For this review, take the finished solid that the model builds, in its own axes (mm). Face numbers are marked on the shaded views. A direction names the side the tool comes from. Coordinates: 2 decimals unless noted, no trailing zeros. Loops run counter-clockwise (first coordinate to the right, second up) from the corner with the lowest first, then second, coordinate; pieces in that order, holes last. Notation, with made-up numbers: (5.5, 83) -> (14.5, 83) arc R26 cw to (14.5, 98) -> close; hole circle Ø1 at (80, 18.25). An arc over 180 degrees is marked (long way). Use a Markdown table: item, result.
from build123d import *

# Parameters (mm, degrees)
F1_DEPTH = 10
F6_DEPTH = 25


with BuildPart() as f1:
    # F0 (on Top) → F1 (new body)
    with BuildSketch(Plane.XY):
        Polygon((25, 4.25), (25, 0), (30, 0), (30, 7.25), (0, 7.25), (0, 4.25), align=None)
    extrude(amount=F1_DEPTH)

    # F2 (on face) → F3 (revolve)
    with BuildSketch(Plane(origin=(0, 7.25, 0), x_dir=(-1, 0, 0), z_dir=(0, 1, 0))):
        with BuildLine():
            Line((-7.5, 7.25), (-7.5, 2.75))
            ThreePointArc((-7.5, 2.75), (-5.25, 5), (-7.5, 7.25))
        make_face()
    revolve(axis=Axis((7.5, 7.25, 5), (0, 0, -1)))

    # F4: F1 across plane


with BuildPart() as f1_1:
    add(f1.part)
    add(f1.part.mirror(Plane.XZ))

    # F5 (on face) → F6 (cut)
    with BuildSketch(Plane.XZ.offset(7.25)):
        with BuildLine():
            ThreePointArc((7.5, 0), (2.5, 5), (7.5, 10))
            Line((7.5, 10), (0, 10))
            Line((0, 10), (0, 0))
            Line((0, 0), (7.5, 0))
        make_face()
    extrude(amount=-F6_DEPTH, mode=Mode.SUBTRACT)


solid = f1_1.part
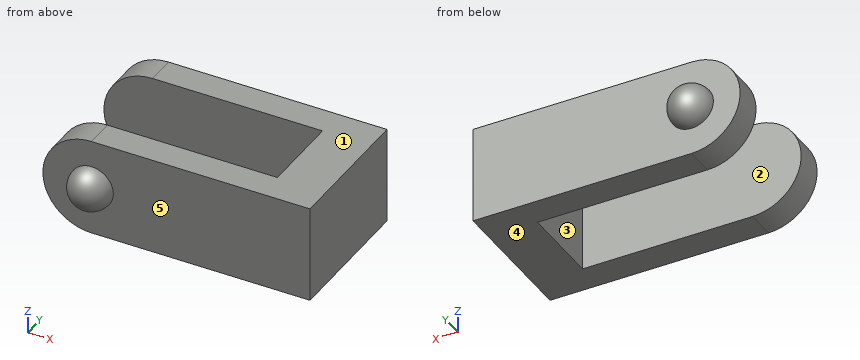
(1) Take a section at B-B on z = 9. Write out the cut boundary in (x, y).
Found:
| item | result |
|---|---|
| outline | (4.5, -7.25) -> (30, -7.25) -> (30, 7.25) -> (4.5, 7.25) -> (4.5, 4.25) -> (25, 4.25) -> (25, -4.25) -> (4.5, -4.25) -> close |
(2) Mouldability with a two-part tool opening along Y and no side actions: class the marked faces 3, 4 and 5 as pulls with the +Y half, pulls with the -Y half, needs draft (parallel to the pull), parting line crosses it, or undercut.
Found:
| item | result |
|---|---|
| face 3 | undercut |
| face 4 | needs draft |
| face 5 | pulls with the -Y half |
(3) Take a section at D-D on y = 2.75. Write out the cut boundary in (x, z).
Found:
| item | result |
|---|---|
| outline | (25, 0) -> (30, 0) -> (30, 10) -> (25, 10) -> close |
(4) For the marked faces 1 and 2, list the 3-axis set-ups (+Z, -Z, +X, -X, +Y, -Y) from which the entire face can be reached by the end or side of a thin tool; tool diameter is ignored.
Found:
| item | result |
|---|---|
| face 1 | +Z, +X, -X, +Y, -Y |
| face 2 | +Z, -Z, -X |
(5) For line 1 along Y through (x, z) = (24.5, 8.25); line 2 along X through (y, z) = (0, 1.5); line 3 along Y through (x, z) = (25.25, 6.5), list the stretches that pass through material, from the lowest coordinate up.
Found:
| item | result |
|---|---|
| line 1 | y = -7.25 to -4.25, 4.25 to 7.25 |
| line 2 | x = 25 to 30 |
| line 3 | y = -7.25 to 7.25 |
(6) Take a section at C-C on x = 5.75. Write out the cut boundary in (y, z).
Found:
| item | result |
|---|---|
| outline | (-7.25, 0.32) -> (-4.25, 0.32) -> (-4.25, 9.68) -> (-7.25, 9.68) -> (-7.25, 6.41) arc R1.41 ccw to (-7.25, 3.59) -> close; (4.25, 0.32) -> (7.25, 0.32) -> (7.25, 3.59) arc R1.41 ccw to (7.25, 6.41) -> (7.25, 9.68) -> (4.25, 9.68) -> close |
(7) For pin 1 Ø1 at (x, z) = (24, 4.5) entering from +Y; pin 2 Ø5 at (x, z) = (11, 6) entering from -Y; pin 3 Ø3 at (x, y) = (15, 1.5) entering from -Z (3 decimals), all flat-tipped, find the tip position at first contact; note any pin that passes through.
Found:
| item | result |
|---|---|
| pin 1 | stops at y = 7.25 |
| pin 2 | stops at y = -9.19 |
| pin 3 | passes through |
(8) Take a section at A-A on x = 19.5. Write out the cut boundary in (y, z).
Found:
| item | result |
|---|---|
| outline | (-7.25, 0) -> (-4.25, 0) -> (-4.25, 10) -> (-7.25, 10) -> close; (4.25, 0) -> (7.25, 0) -> (7.25, 10) -> (4.25, 10) -> close |
